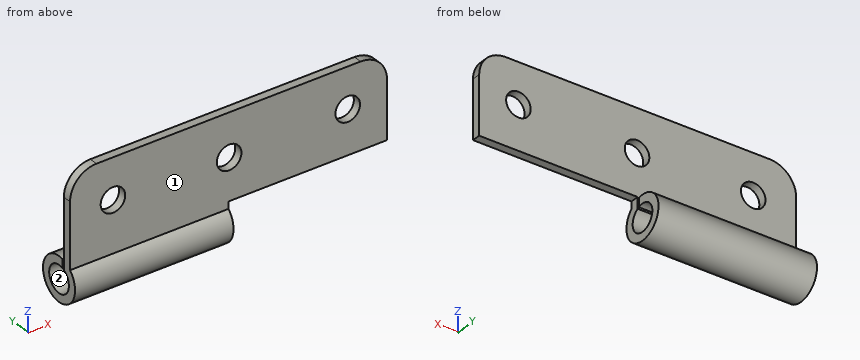
```python
from build123d import *

# Parameters (mm, degrees)
SKETCH_1_R               = 4.15
EXTRUDE_1_DEPTH          = 60
SKETCH_2_R               = 2.325
EXTRUDE_2_DEPTH          = 1.6
FILLET_1_R               = 5
CUT_EXTRUDE_2_DEPTH      = 64.492873616
CUT_EXTRUDE_1_DEPTH      = 64.586810739
CUT_EXTRUDE_1_DEPTH_BACK = 64.586810739
SKETCH_4_W               = 30
SKETCH_4_H               = 8.5


with BuildPart() as part:
    # Эскиз1 → Бобышка-Вытянуть1 (new body)
    with BuildSketch(Plane(origin=(0, 0, 0), x_dir=(0, 0, -1), z_dir=(1, 0, 0))):
        Circle(SKETCH_1_R)
    extrude(amount=EXTRUDE_1_DEPTH)

    # Эскиз2 → Бобышка-Вытянуть2 (add)
    with BuildSketch(Plane(origin=(0, -2.85, 0), x_dir=(1, 0, 0), z_dir=(0, 1, 0))):
        Polygon((0, -4.15), (0, -20.35), (60, -20.35), (60, -4.15), (60, 0), (0, 0), align=None)
        with Locations(Location((8.125, -12.675, 0), (0, 0, 270))):
            Circle(SKETCH_2_R, mode=Mode.SUBTRACT)
        with Locations(Location((30.119163283, -12.225, 0), (0, 0, 270))):
            Circle(SKETCH_2_R, mode=Mode.SUBTRACT)
        with Locations(Location((52.569163283, -12.675, 0), (0, 0, 270))):
            Circle(SKETCH_2_R, mode=Mode.SUBTRACT)
    extrude(amount=EXTRUDE_2_DEPTH)

    # Скругление1
    fillet_1_edges = [part.edges().sort_by_distance(p)[0] for p in [
        (0, -2.05, 20.35),
        (60, -2.05, 20.35),
    ]]
    fillet(fillet_1_edges, radius=FILLET_1_R)

    # Эскиз5 → Вырез-Вытянуть2 (cut, through all)
    with BuildSketch(Plane.ZY):
        with BuildLine():
            Line((3.957271787, -1.25), (2.222611077, -1.25))
            ThreePointArc((2.222611077, -1.25), (-2.299419251, 1.102347998), (2.366431913, -0.95))
            Line((2.366431913, -0.95), (4.039801975, -0.95))
            Line((4.039801975, -0.95), (4.039801975, -1.25))
            Line((4.039801975, -1.25), (3.957271787, -1.25))
        make_face()
    extrude(amount=-CUT_EXTRUDE_2_DEPTH, mode=Mode.SUBTRACT)

    # Эскиз4 → Вырез-Вытянуть1 (cut, two sides: drawn at the far end of the back side and taken through both)
    with BuildSketch(Plane(origin=(0, -1.25, 0), x_dir=(1, 0, 0), z_dir=(0, 1, 0)).offset(-CUT_EXTRUDE_1_DEPTH_BACK)):
        with Locations((45, -0.1)):
            Rectangle(SKETCH_4_W, SKETCH_4_H)
    extrude(amount=CUT_EXTRUDE_1_DEPTH + CUT_EXTRUDE_1_DEPTH_BACK, mode=Mode.SUBTRACT)


solid = part.part
```
Can you work these out from the model? Positions are in its coordinate system, mm. Face numbers are marked on the shaded views. Round coordinates to 2 decimals unless told otherwise and drop trailing zeros. Loops run counter-clockwise (first coordinate to the right, second up) from the corner with the lowest first, then second, coordinate; pieces in that order, holes last. Notation, with made-up numbers: (-39, 37.25) -> (4, 37.25) arc R31 ccw to (4, 70.25) -> close; hole circle Ø1 at (67.5, 54.25). An arc over 180 degrees is marked (long way). One line per item, written item: value. Start each with the question number.
1. If we section it at C-C, the plane z = 11.75: Write out the boundary of the cut face in (x, y).
2. If we section it at D-D, the plane x = 26.5: Write out the boundary of the cut face in (y, z), then the cut area to 3 significant figures.
3. If I drill on probe 1 along Z at (x, y) = (12.5, -0.25); probe 2 along Z at (x, y) = (12.5, -1.5); probe 3 along Y at (x, z) = (39.5, 19.25), over which ranges is the centre line in solid material (lowest first)?
4. If we mould it in two halves opening along Y, with no side actions, what happens to the marked faces 1 and 2? For each: pulls with the +Y half, pulls with the -Y half, needs draft (parallel to the pull), parting line crosses it, or undercut.
5. If we section it at A-A, the plane y = 0: Write out the boundary of the cut face in (x, z), then the cut area to 3 significant figures.
6. For pin 1 (1 mm diameter, centred on x = 9, z = 3.5, fed in from +Y); pin 2 (0.8 mm diameter, centred on x = 50, y = -2.5, fed in from -Z); pin 3 (5.5 mm diameter, centred on x = 8.125, z = 12.675, fed in from +Y); pin 4 (3 mm diameter, centred on x = 43, z = 1, fed in from +Y), each with a flat end and sliding along its axis, tell me the tip position at first contact or that it passes through.
Calculated:
1. outline: (0, -2.85) -> (5.99, -2.85) -> (5.99, -1.25) -> (0, -1.25) -> close; (10.26, -2.85) -> (27.84, -2.85) -> (27.84, -1.25) -> (10.26, -1.25) -> close; (32.4, -2.85) -> (50.44, -2.85) -> (50.44, -1.25) -> (32.4, -1.25) -> close; (54.7, -2.85) -> (60, -2.85) -> (60, -1.25) -> (54.7, -1.25) -> close
2. outline: (-2.85, 3.02) arc R4.15 ccw (long way) to (-0.95, 4.04) -> (-0.95, 2.37) arc R2.55 cw (long way) to (-1.25, 2.22) -> (-1.25, 20.35) -> (-2.85, 20.35) -> close
2. area: 60.0 mm²
3. probe 1: z = -4.14 to -2.54, 2.54 to 4.14
3. probe 2: z = -3.87 to -2.06, 2.06 to 20.35
3. probe 3: y = -2.85 to -1.25
4. face 1: pulls with the -Y half
4. face 2: undercut
5. outline: (0, -4.15) -> (30, -4.15) -> (30, -2.55) -> (0, -2.55) -> close; (0, 2.55) -> (30, 2.55) -> (30, 4.15) -> (0, 4.15) -> close
5. area: 96.0 mm²
6. pin 1: stops at y = 2.87
6. pin 2: stops at z = 4.35
6. pin 3: stops at y = -1.25
6. pin 4: passes through
